```python
from build123d import *

# Parameters (mm, degrees)
BOSS_EXTRUDE1_DEPTH = 0.75
FILLET1_R           = 1.8
CUT_EXTRUDE3_DEPTH  = 36.680336791
SKETCH5_R           = 1.6
CUT_EXTRUDE4_DEPTH  = 20.5
LPATTERN1_COUNT     = 12
LPATTERN1_PITCH     = 2.85
SKETCH8_R           = 1.5
CUT_EXTRUDE5_DEPTH  = 20.5
CUT_REVOLVE1_ANGLE  = 90


with BuildPart() as part:
    # Sketch1 → Boss-Extrude1 (new, symmetric)
    with BuildSketch(Plane.XY):
        with BuildLine():
            Line((0, 6.712848625), (0, 3))
            Line((0, 3), (34.384210526, 1.3))
            Line((34.384210526, 1.3), (30.5, 9.5))
            Line((30.5, 9.5), (8.534429687, 9.5))
            ThreePointArc((8.534429687, 9.5), (7.017751028, 9.384315143), (5.53616372, 9.039937169))
            Line((5.53616372, 9.039937169), (0.560138723, 7.476043599))
            ThreePointArc((0.560138723, 7.476043599), (0.155062398, 7.186193625), (0, 6.712848625))
        make_face()
        with BuildLine():
            Line((30.5, 9.5), (34.384210526, 1.3))
            Line((34.384210526, 1.3), (35, 0))
            Line((35, 0), (47, 0))
            Line((47, 0), (47, 8))
            Line((47, 8), (41, 8))
            ThreePointArc((41, 8), (40.646446609, 8.146446609), (40.5, 8.5))
            Line((40.5, 8.5), (40.5, 9))
            ThreePointArc((40.5, 9), (40.353553391, 9.353553391), (40, 9.5))
            Line((40, 9.5), (30.5, 9.5))
        make_face()
    extrude(amount=BOSS_EXTRUDE1_DEPTH, both=True)

    # Fillet1
    fillet1_edges = [part.edges().sort_by_distance(p)[0] for p in [
        (47, 8, 0),
        (47, 0, 0),
    ]]
    fillet(fillet1_edges, radius=FILLET1_R)

    # Sketch4 → Cut-Extrude3 (cut, through all)
    with BuildSketch(Plane(origin=(34.384210526, 0, 0), x_dir=(0, 0, -1), z_dir=(1, 0, 0))):
        Polygon((-0.75, 1.3), (-0.125, 1.3), (-0.75, 7), align=None)
        Polygon((0.75, 1.3), (0.125, 1.3), (0.75, 7), align=None)
    extrude(amount=-CUT_EXTRUDE3_DEPTH, mode=Mode.SUBTRACT)

    # Sketch5 → Cut-Extrude4 (cut, along a direction that is not the sketch's normal)
    with BuildSketch(Plane(origin=(0, 0.001900815, 0.017335437), x_dir=(-1, 0, 0), z_dir=(0, -0.10899585570756742, -0.9940422040530147))):
        with Locations((-32.784210526, 0.634532433)):
            Circle(SKETCH5_R)
    cut_extrude4 = extrude(amount=-CUT_EXTRUDE4_DEPTH, dir=(0, 0.6987711700907747, -0.7153452675806066), mode=Mode.SUBTRACT)

    # LPattern1: Cut-Extrude4 ×12
    with Locations(*[Vector(-0.998765374567026, 0.049380256541427955, -0.005414501813753065) * (i * LPATTERN1_PITCH) for i in range(1, LPATTERN1_COUNT)]):
        add(cut_extrude4, mode=Mode.SUBTRACT)

    # Sketch8 → Cut-Extrude5 (cut)
    with BuildSketch(Plane.XY.offset(0.75)):
        with Locations((43.1, 4)):
            Circle(SKETCH8_R)
    extrude(amount=-CUT_EXTRUDE5_DEPTH, mode=Mode.SUBTRACT)

    # Sketch2 → Cut-Revolve1 (revolve, cut)
    with BuildSketch(Plane(origin=(0, 0, -0.75), x_dir=(-1, 0, 0), z_dir=(0, 0, -1))):
        with BuildLine():
            Line((-30.5, 8.5), (-16.5, 8.5))
            ThreePointArc((-16.5, 8.5), (-23.5, 7.699337741), (-30.5, 8.5))
        make_face()
    revolve(axis=Axis((30.5, 8.5, -0.75), (-1, 0, 0)), revolution_arc=CUT_REVOLVE1_ANGLE, mode=Mode.SUBTRACT)


solid = part.part
```
Geometry: final body of the model. Coordinates: model frame, mm. A direction names the side the tool comes from. Round coordinates to 2 decimals unless told otherwise and drop trailing zeros. Order: outer loops, then holes, each group sorted by start corner. A loop starts at its lowest first (then second) coordinate and runs counter-clockwise, first axis right, second up. Notation, with made-up numbers: M 32,51.25 L 56,51.25 A19 ccw 56,78.25 Z; hole C -2.75,29 d3. An arc over 180 degrees is marked long. One line per item, written item: value.
(1) Cut plane A-A (x = 44). Return the cut outline in (y, z), and give its area (3 significant figures).
Result sheet:
outline: M 0,-0.75 L 2.8,-0.75 L 2.8,0.75 L 0,0.75 Z; M 5.2,-0.75 L 8,-0.75 L 8,0.75 L 5.2,0.75 Z
area: 8.40 mm2
(2) Line query: probe 1 along Y at (x, z) = (43.1, 0.2); probe 2 along Y at (x, z) = (43.5, -0.05); probe 3 along Z at (x, y) = (11, 3). Output: solid intervals per line, ascending. Write a range as [from, to].
Result sheet:
probe 1: [0, 2.5], [5.5, 8]
probe 2: [0, 2.55], [5.45, 8]
probe 3: [-0.3, 0.31]
(3) Reachability of faces 1 (the flat face through (43, 8, 0)), 2 (the flat face through (17.433, 4.743, 0.503)), 3 (the flat face through (17.433, 4.743, -0.503)) from +Z, -Z, +X, -X, +Y, -Y: full face, straight path, thin tool, end or side. Return the list, or none.
Result sheet:
face 1: +Z, -Z, +X, +Y
face 2: +Z, -X, -Y
face 3: -Z, -X, -Y
(4) Pin query (flat end, axial travel): P1, Ø0.8, axis at x = 42.5, z = 0, coming from the +Y side. Return the tip coordinate at first contact, or that it passes through.
Result sheet:
P1: y = 8
(5) Pull-direction query (Y, two-part tool) for faces 4 (the flat face through (30, 8, 0.75)), 5 (the flat face through (34.688, 0.659, 0.01)), 6 (the flat face through (23.4, 8.5, -0.4)); classes: pulls with the +Y half, pulls with the -Y half, needs draft (parallel to the pull), parting line crosses it, or undercut.
Result sheet:
face 4: needs draft
face 5: pulls with the -Y half
face 6: undercut
